Check sheet for the drawn part. Datum: minimum x, y, z corner. Units: mm. Coordinates: 2 decimals unless noted, no trailing zeros. Write each loop counter-clockwise with the first axis right and the second up, starting at its lowest first coordinate (ties: lowest second). Pieces come first, ordered by that corner, then holes. Notation, with made-up numbers: (42, 68) - (62, 68) arc R24 ccw to (62, 102) - close; hole circle Ø4 at (-28, 28). An arc over 180 degrees is marked (long way). Use one line per item in the form item = value. Start each with the question number.
1. Cross-section at D-D on y = 8. Record the boundary of the cut face in (x, z).
2. Scan lines: line 1 along Y through (x, z) = (7.5, 3.75); line 2 along X through (y, z) = (2.25, 7.25); line 3 along Y through (x, z) = (12.75, 6.5) (1 decimal). Record each from-to range of solid material in increasing order.
3. Cross-section at B-B on z = 7.25. Record the boundary of the cut face in (x, y), then the cut area to 3 significant figures.
4. Cross-section at C-C on x = 7.5. Record the boundary of the cut face in (y, z).
5. Draft check along Y on the marked faces 1, 2 and 3. Enter one of: +Y half, -Y half, draft (parallel to the pull), parting line (faces both ways), or undercut.
6. Cross-section at A-A on y = 3. Record the boundary of the cut face in (x, z).
7. Go/stop test with a flat-tipped pin: pin 1 Ø2 at (x, y) = (13, 7.5) entering from -Z. Record where the tip stops, or that it passes through.
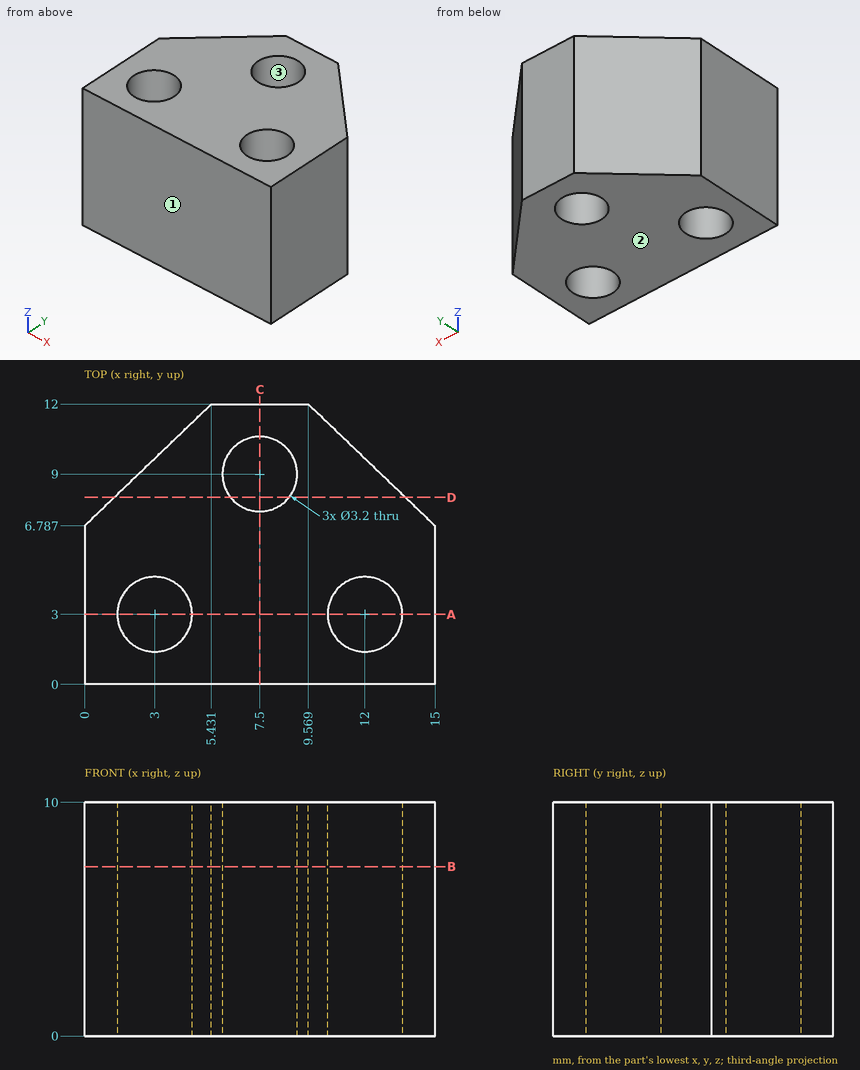
Final values:
q1.outline = (1.26, 0) - (6.25, 0) - (6.25, 10) - (1.26, 10) - close; (8.75, 0) - (13.74, 0) - (13.74, 10) - (8.75, 10) - close
q2.line_1 = 0 to 7.4, 10.6 to 12
q2.line_2 = 0 to 1.59, 4.41 to 10.59, 13.41 to 15
q2.line_3 = 0 to 1.6, 4.4 to 8.9
q3.outline = (0, 0) - (15, 0) - (15, 6.79) - (9.57, 12) - (5.43, 12) - (0, 6.79) - close; hole circle Ø3.2 at (3, 3); hole circle Ø3.2 at (7.5, 9); hole circle Ø3.2 at (12, 3)
q3.area = 128 mm²
q4.outline = (0, 0) - (7.4, 0) - (7.4, 10) - (0, 10) - close; (10.6, 0) - (12, 0) - (12, 10) - (10.6, 10) - close
q5.face_1 = -Y half
q5.face_2 = draft
q5.face_3 = undercut
q6.outline = (0, 0) - (1.4, 0) - (1.4, 10) - (0, 10) - close; (4.6, 0) - (10.4, 0) - (10.4, 10) - (4.6, 10) - close; (13.6, 0) - (15, 0) - (15, 10) - (13.6, 10) - close
q7.pin_1 = 0
